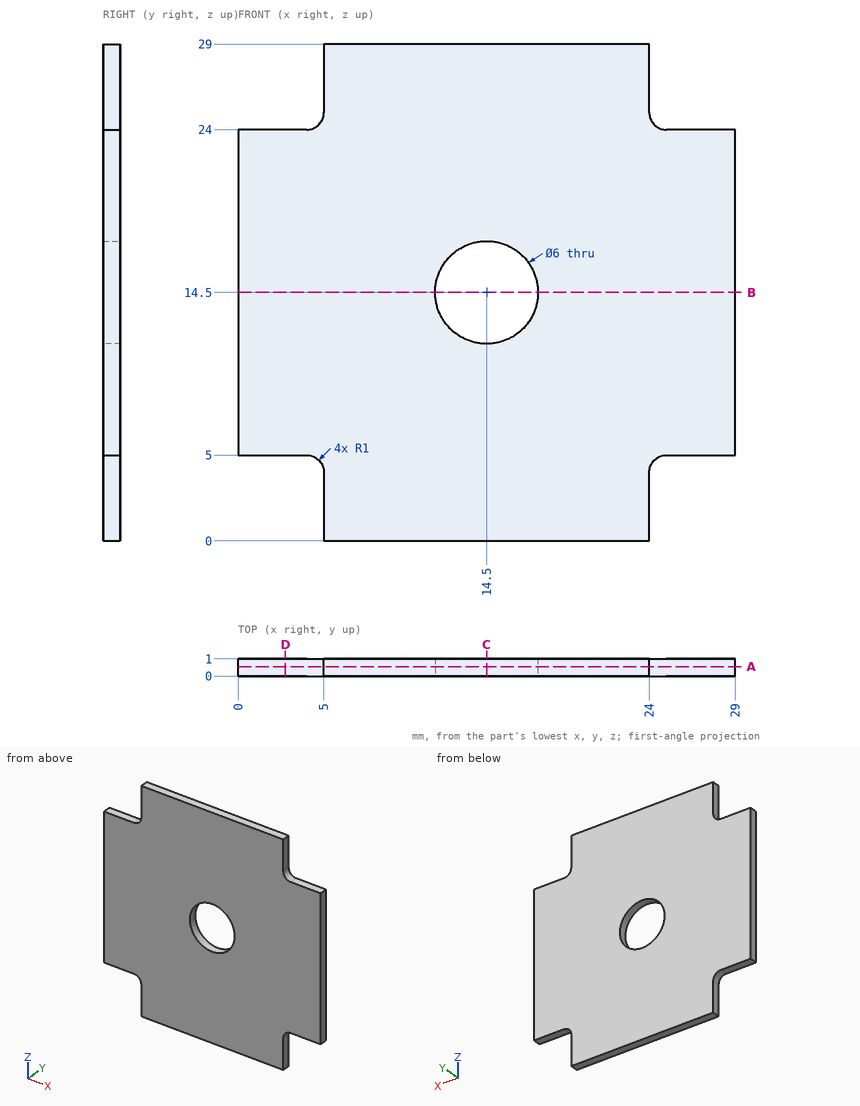
Design review of the part shown in the three views and the two pictorial views. Dimensions are in mm from the part's minimum x, y and z. Round coordinates to 2 decimals unless told otherwise and drop trailing zeros. Loops run counter-clockwise (first coordinate to the right, second up) from the corner with the lowest first, then second, coordinate; pieces in that order, holes last. Notation, with made-up numbers: (34.25, 71.25) -> (71.25, 71.25) arc R18 cw to (71.25, 104.25) -> close; hole circle Ø5 at (42.5, 62.25). An arc over 180 degrees is marked (long way). Use one line per item in the form item = value. Start each with the question number.
Q1. We need section B-B on z = 14.5. Give the boundary of the cut face in (x, y), then the cut area to 3 significant figures.
Q2. Wall thickness on line 1 along X through (y, z) = (0.65, 14.5); line 2 along Z through (x, y) = (2, 0.65); line 3 along X through (y, z) = (0.7, 16.75): over which ranges is each line inside the solid? List them lowest first. Write a range as [from, to].
Q3. We need section C-C on x = 14.5. Give the boundary of the cut face in (y, z), then the cut area to 3 significant figures.
Q4. We need section D-D on x = 2.75. Give the boundary of the cut face in (y, z).
Q5. We need section A-A on y = 0.55. Give the boundary of the cut face in (x, z).
Q6. For pin 1 Ø0.5 at (y, z) = (0.5, 2.5) entering from -X; pin 2 Ø0.5 at (x, y) = (27, 0.5) entering from -Z; pin 3 Ø0.5 at (x, y) = (1, 0.5) entering from +Z, all flat-tipped, find the tip position at first contact; note any pin that passes through.
Calculated:
q1.outline = (0, 0) -> (11.5, 0) -> (11.5, 1) -> (0, 1) -> close; (17.5, 0) -> (29, 0) -> (29, 1) -> (17.5, 1) -> close
q1.area = 23.0 mm²
q2.line_1 = [0, 11.5], [17.5, 29]
q2.line_2 = [5, 24]
q2.line_3 = [0, 12.52], [16.48, 29]
q3.outline = (0, 0) -> (1, 0) -> (1, 11.5) -> (0, 11.5) -> close; (0, 17.5) -> (1, 17.5) -> (1, 29) -> (0, 29) -> close
q3.area = 23.0 mm²
q4.outline = (0, 5) -> (1, 5) -> (1, 24) -> (0, 24) -> close
q5.outline = (0, 5) -> (4, 5) arc R1 cw to (5, 4) -> (5, 0) -> (24, 0) -> (24, 4) arc R1 cw to (25, 5) -> (29, 5) -> (29, 24) -> (25, 24) arc R1 cw to (24, 25) -> (24, 29) -> (5, 29) -> (5, 25) arc R1 cw to (4, 24) -> (0, 24) -> close; hole circle Ø6 at (14.5, 14.5)
q6.pin_1 = 5
q6.pin_2 = 5
q6.pin_3 = 24
